Verification items for the finished model (mm, model axes). A direction names the side the tool comes from. Give positions to 0.01 mm unless a question says otherwise; leave off trailing zeros. Write each loop counter-clockwise with the first axis right and the second up, starting at its lowest first coordinate (ties: lowest second). Pieces come first, ordered by that corner, then holes. Notation, with made-up numbers: M -0.75,69 L 44.25,69 A8 cw 44.25,79 Z; hole C -23.5,3 d2. An arc over 180 degrees is marked long. Write item = value, one per line.
from build123d import *

# Parameters (mm, degrees)
SKETCH1_W           = 20
SKETCH1_H           = 12.6
BOSS_EXTRUDE1_DEPTH = 5
CUT_EXTRUDE1_REACH  = 19.616
SKETCH2_W           = 20
SKETCH2_H           = 0.5
CUT_EXTRUDE2_REACH  = 89.84
SKETCH3_W           = 20
SKETCH3_H           = 2
BOSS_EXTRUDE2_DEPTH = 10.6
CUT_EXTRUDE4_DEPTH  = 88.839697745
FILLET1_R           = 3
CUT_EXTRUDE5_DEPTH  = 3
CHAMFER2_SIZE       = 1
FILLET2_R           = 2


with BuildPart() as part:
    # Sketch1 → Boss-Extrude1 (new body)
    with BuildSketch(Plane.XY):
        with Locations((-1.25, 80.7)):
            Rectangle(SKETCH1_W, SKETCH1_H)
    extrude(amount=BOSS_EXTRUDE1_DEPTH)

    # Sketch2 → Cut-Extrude1 (cut, up to next)
    with BuildSketch(Plane(origin=(0, 87, 0), x_dir=(1, 0, 0), z_dir=(0, 1, 0)), mode=Mode.PRIVATE) as cut_extrude1_sk1:
        with Locations((-1.25, -0.25)):
            Rectangle(SKETCH2_W, SKETCH2_H)
    cut_extrude1_tool1 = extrude(cut_extrude1_sk1.sketch, amount=-CUT_EXTRUDE1_REACH, mode=Mode.PRIVATE) & part.part
    add(cut_extrude1_tool1.solids().sort_by_distance((-1.25, 87, 0.25))[0], mode=Mode.SUBTRACT)

    # Sketch3 → Cut-Extrude2 (cut, up to next)
    with BuildSketch(Plane.XY.offset(5), mode=Mode.PRIVATE) as cut_extrude2_sk1:
        with Locations((-1.25, 75.4)):
            Rectangle(SKETCH3_W, SKETCH3_H)
    cut_extrude2_tool1 = extrude(cut_extrude2_sk1.sketch, amount=-CUT_EXTRUDE2_REACH, mode=Mode.PRIVATE) & part.part
    add(cut_extrude2_tool1.solids().sort_by_distance((-1.25, 75.4, 5))[0], mode=Mode.SUBTRACT)

    # Sketch4 → Boss-Extrude2 (add)
    with BuildSketch(Plane(origin=(0, 87, 0), x_dir=(1, 0, 0), z_dir=(0, 1, 0))):
        Polygon((-4.884848004, -0.5), (-3.634848004, 0.75), (1.134848004, 0.75), (2.384848004, -0.5), align=None)
    extrude(amount=-BOSS_EXTRUDE2_DEPTH)

    # Sketch6 → Cut-Extrude4 (cut, symmetric)
    with BuildSketch(Plane(origin=(0, 0, 0.5), x_dir=(-1, 0, 0), z_dir=(0, 0, -1))):
        with BuildLine():
            Line((-6.317424002, 82.75), (-4.817424002, 82.75))
            ThreePointArc((-4.817424002, 82.75), (-3.767424002, 81.7), (-4.817424002, 80.65))
            Line((-4.817424002, 80.65), (-6.317424002, 80.65))
            ThreePointArc((-6.317424002, 80.65), (-7.367424002, 81.7), (-6.317424002, 82.75))
        make_face()
    cut_extrude4 = extrude(amount=CUT_EXTRUDE4_DEPTH, both=True, mode=Mode.SUBTRACT)

    # Fillet1
    fillet1_edges = [part.edges().sort_by_distance(p)[0] for p in [
        (-11.25, 87, 2.75),
        (-11.25, 76.4, 2.75),
        (8.75, 76.4, 2.75),
        (8.75, 87, 2.75),
    ]]
    fillet(fillet1_edges, radius=FILLET1_R)

    # Sketch7 → Cut-Extrude5 (cut)
    with BuildSketch(Plane.XY.offset(5)):
        with BuildLine():
            Line((6.25, 79.7), (4.884848004, 79.7))
            ThreePointArc((4.884848004, 79.7), (2.884848004, 81.7), (4.884848004, 83.7))
            Line((4.884848004, 83.7), (6.25, 83.7))
            ThreePointArc((6.25, 83.7), (8.25, 81.7), (6.25, 79.7))
        make_face()
    cut_extrude5 = extrude(amount=-CUT_EXTRUDE5_DEPTH, mode=Mode.SUBTRACT)

    # Mirror1: Cut-Extrude4, Cut-Extrude5 across plane
    add(cut_extrude4.mirror(Plane(origin=(-1.25, 0, 0), x_dir=(0, 0, 1), z_dir=(1, 0, 0))), mode=Mode.SUBTRACT)
    add(cut_extrude5.mirror(Plane(origin=(-1.25, 0, 0), x_dir=(0, 0, 1), z_dir=(1, 0, 0))), mode=Mode.SUBTRACT)

    # Chamfer2
    # the kernel refuses this chamfer: 1 mm, written as the material it takes off along each edge
    with BuildSketch(Plane(origin=(5.75, 76.4, 5), x_dir=(0, -0.02749587661058217, -0.9996219169112968), z_dir=(-1, 0, 0)), Plane(origin=(-8.25, 87, 5), x_dir=(0, 0.02749587661058217, -0.9996219169112968), z_dir=(1, 0, 0))) as chamfer2_piece_1:
        Polygon((CHAMFER2_SIZE * 0.999621916911, -CHAMFER2_SIZE * 0.0274958766106), (-CHAMFER2_SIZE * 0.0274958766106, -CHAMFER2_SIZE * 0.999621916911), (0, 0), align=None)
    extrude(amount=14, mode=Mode.SUBTRACT)
    with BuildSketch(Plane(origin=(8.75, 84, 5), x_dir=(-0.9996219169112968, 0, 0.02749587661058651), z_dir=(0, -1, 0))) as chamfer2_piece_2:
        Polygon((CHAMFER2_SIZE * 0.999621916911, CHAMFER2_SIZE * 0.0274958766106), (-CHAMFER2_SIZE * 0.0274958766106, CHAMFER2_SIZE * 0.999621916911), (0, 0), align=None)
    extrude(amount=4.6, mode=Mode.SUBTRACT)
    with BuildSketch(Plane(origin=(-11.25, 79.4, 5), x_dir=(-0.027495876610585623, 0, -0.9996219169112968), z_dir=(0, 1, 0))) as chamfer2_piece_3:
        Polygon((CHAMFER2_SIZE * 0.999621916911, -CHAMFER2_SIZE * 0.0274958766106), (-CHAMFER2_SIZE * 0.0274958766106, -CHAMFER2_SIZE * 0.999621916911), (0, 0), align=None)
    extrude(amount=4.6, mode=Mode.SUBTRACT)
    with BuildSketch(Plane(origin=(5.75, 84, 5), x_dir=(0, 1, 0), z_dir=(-1, 0, 0))) as chamfer2_piece_4:
        Polygon((3 - CHAMFER2_SIZE, 0), (3, CHAMFER2_SIZE), (3, 0), align=None)
    revolve(axis=Axis((5.75, 84, 5), (0, 0, -1)), revolution_arc=90, mode=Mode.SUBTRACT)
    with BuildSketch(Plane(origin=(-8.25, 84, 5), x_dir=(0, 1, 0), z_dir=(1, 0, 0))) as chamfer2_piece_5:
        Polygon((3, -CHAMFER2_SIZE), (3 - CHAMFER2_SIZE, 0), (3, 0), align=None)
    revolve(axis=Axis((-8.25, 84, 5), (0, 0, 1)), revolution_arc=90, mode=Mode.SUBTRACT)
    with BuildSketch(Plane(origin=(-8.25, 79.4, 5), x_dir=(0, -1, 0), z_dir=(1, 0, 0))) as chamfer2_piece_6:
        Polygon((3, CHAMFER2_SIZE), (3 - CHAMFER2_SIZE, 0), (3, 0), align=None)
    revolve(axis=Axis((-8.25, 79.4, 5), (0, 0, -1)), revolution_arc=90, mode=Mode.SUBTRACT)
    with BuildSketch(Plane(origin=(5.75, 79.4, 5), x_dir=(0, -1, 0), z_dir=(-1, 0, 0))) as chamfer2_piece_7:
        Polygon((3 - CHAMFER2_SIZE, 0), (3, -CHAMFER2_SIZE), (3, 0), align=None)
    revolve(axis=Axis((5.75, 79.4, 5), (0, 0, 1)), revolution_arc=90, mode=Mode.SUBTRACT)

    # Fillet2
    fillet2_edges = [part.edges().sort_by_distance(p)[0] for p in [
        (2.384848004, 81.7, 0.5),
        (-4.884848004, 81.7, 0.5),
        (-3.634848004, 81.7, -0.75),
        (1.134848004, 81.7, -0.75),
    ]]
    fillet(fillet2_edges, radius=FILLET2_R)


solid = part.part
1) Cross-section at B-B on y = 82.5. Record the boundary of the cut face in (x, z).
From the geometry:
outline = M -11.25,0.5 L -9.5,0.5 L -9.5,2 L -10.58,2 L -10.58,4.67 L -11.25,4 Z; M -6.64,0.5 L -5.71,0.5 A2 cw -4.3,-0.09 L -4.22,-0.16 A2 ccw -2.81,-0.75 L 0.31,-0.75 A2 ccw 1.72,-0.16 L 1.8,-0.09 A2 cw 3.21,0.5 L 4.14,0.5 L 4.14,2 L 3.05,2 L 3.05,5 L -5.55,5 L -5.55,2 L -6.64,2 Z; M 7,0.5 L 8.75,0.5 L 8.75,4 L 8.08,4.67 L 8.08,2 L 7,2 Z
2) Tool access check on faces 4 (the cylindrical face through (8.25, 81.74, 3.52)), 5 (the flat face through (6, 80.65, 1)), 6 (the conical face through (-9.916, 77.697, 4.618)). Record the directions out of +Z, -Z, +X, -X, +Y, -Y that give a thin tool (end or side, any length) a straight path to the whole face; none if there is none.
From the geometry:
face_4 = +Z
face_5 = +Z, -Z
face_6 = +Z, -X, -Y
3) Depth check by flat-ended pin: P1, Ø1, axis at x = 2.5, y = 78, coming from the -Z side; P2, Ø1, axis at x = -8, y = 80.5, coming from the +Z side; P3, Ø1.7, axis at x = -8, y = 81, coming from the -Z side; P4, Ø1.6, axis at x = -8.5, z = 1, coming from the -Y side. Enter the tip coordinate at first touch or a pass-through.
From the geometry:
P1 = 0.09
P2 = 2
P3 = 0.5
P4 = 76.4
4) Cross-section at A-A on z = 1.8. Record the boundary of the cut face in (x, y), plus the area to 3 significant figures.
From the geometry:
outline = M -11.25,79.4 A3 ccw -8.25,76.4 L 5.75,76.4 A3 ccw 8.75,79.4 L 8.75,84 A3 ccw 5.75,87 L -8.25,87 A3 ccw -11.25,84 Z; hole M -8.82,80.65 L -7.32,80.65 A1.05 ccw -7.32,82.75 L -8.82,82.75 A1.05 ccw Z; hole M 4.82,80.65 L 6.32,80.65 A1.05 ccw 6.32,82.75 L 4.82,82.75 A1.05 ccw Z
area = 191 mm^2
5) Cross-section at D-D on z = 2.65. Record the boundary of the cut face in (x, y), plus the area to 3 significant figures.
From the geometry:
outline = M -11.25,79.4 A3 ccw -8.25,76.4 L 5.75,76.4 A3 ccw 8.75,79.4 L 8.75,84 A3 ccw 5.75,87 L -8.25,87 A3 ccw -11.25,84 Z; hole M -8.75,79.7 L -7.38,79.7 A2 ccw -7.38,83.7 L -8.75,83.7 A2 ccw Z; hole M 4.88,79.7 L 6.25,79.7 A2 ccw 6.25,83.7 L 4.88,83.7 A2 ccw Z
area = 168 mm^2
6) Material ranges on probe 1 along X at (y, z) = (80.5, 4.7); probe 2 along X at (y, z) = (82.5, 1.2); probe 3 along X at (y, z) = (77.75, 3.55), recorded low to high. Write a range as from..to.
From the geometry:
probe_1 = -10.55..-10.35, -5.78..3.28, 7.85..8.05
probe_2 = -11.25..-9.5, -6.64..4.14, 7..8.75
probe_3 = -10.76..8.26
7) Cross-section at C-C on x = -6. Record the boundary of the cut face in (y, z).
From the geometry:
outline = M 76.4,0.5 L 87,0.5 L 87,4 L 86,5 L 83.14,5 L 83.14,2 L 80.26,2 L 80.26,5 L 77.4,5 L 76.4,4 Z
8) Draft check along Y on faces 1 (the flat face through (-11.25, 82, 2)), 2 (the cylindrical face through (-5.385, 81.656, 3.521)), 3 (the flat face through (-1.2, 76.9, 4.5)). Enter one of: +Y half, -Y half, draft (parallel to the pull), parting line (faces both ways), or undercut.
From the geometry:
face_1 = draft
face_2 = undercut
face_3 = -Y half
